Work out the finished part from the listing and answer in its coordinate system (mm). A direction names the side the tool comes from. Give positions to 0.01 mm unless a question says otherwise; leave off trailing zeros. Write each loop counter-clockwise with the first axis right and the second up, starting at its lowest first coordinate (ties: lowest second). Pieces come first, ordered by that corner, then holes.
1) A tool of negligible diameter and unlimited length cuts with its end or side. For faces 5 (the face through (49, 166, 5.5)), 6 (the face through (110, 170, 3)), 7 (the face through (-10, 170, 3)), from which of +Z, -Z, +X, -X, +Y, -Y can it reach the whole face along a straight path? Write none if from no direction.
2) Find section D-D (x = 18). Determine the outline of the cut face in (y, z), plus the area to 3 significant figures.
3) Find section B-B (y = 176.5). Determine the outline of the cut face in (x, z), plus the area to 3 significant figures.
4) Straight lines are drawn through the part: probe 1 along Y at (x, z) = (105, 2.95); probe 2 along X at (y, z) = (186, 1.65); probe 3 along X at (y, z) = (183, 3.4). For each, find the intervals that lie inside material, in ascending order.
5) Find section C-C (x = 50). Determine the outline of the cut face in (y, z).
6) Find section A-A (z = 3.95). Determine the outline of the cut face in (x, y), plus the area to 3 significant figures.
7) Determine the mould class of faces 1 (the face through (49, 166, 0)), 2 (the face through (100, 188, 3)), 3 (the face through (50.82, 170.01, 2.71)), 4 (the face through (-20, 160, 3)) for opening direction X: pulls with the +X half, pulls with the -X half, needs draft (parallel to the pull), parting line crosses it, or undercut.
8) Given pin 1 Ø1.5 at (x, y) = (83.5, 162.5) entering from -Z; pin 2 Ø1.5 at (y, z) = (177, 1) entering from -X, each flat-ended and moving along its own axis, determine where each tip first touches the part or whether it passes through.
Autodesk Inventor part; units mm, degrees
ref_plane "YZ Plane" through (0, 0, 0) normal (1, 0, 0) x (0, 1, 0)
ref_plane "XZ Plane" through (0, 0, 0) normal (0, 1, 0) x (-1, 0, 0)
ref_plane "XY Plane" through (0, 0, 0) normal (0, 0, 1) x (1, 0, 0)
sketch "Sketch1" plane through (0, 0, 0) normal (0, 0, 1) x (1, 0, 0)
  line L0 (0, 170) -> (100, 170)
  circle A0 centre (50, 207.5) radius 37.5
  line L1 (100, 150) -> (0, 150)
  line L2 (120, 170) -> (-20, 170)
  line L3 (100, 170) -> (100, 207.5)
  line L4 (100, 207.5) -> (87.5, 207.5)
  line L5 (0, 170) -> (0, 207.5)
  line L6 (0, 207.5) -> (12.5, 207.5)
  line L7 (-20, 170) -> (-20, 150)
  line L8 (-20, 150) -> (0, 150)
  line L9 (100, 150) -> (120, 150)
  line L10 (120, 150) -> (120, 170)
  point P0 (0, 0)
  dimension "d0" = 75
  dimension "d1" = 140
extrude "Extrusion1" add sketch "Sketch1" along normal blind 5.5 contours L5 L6 A0 L0 | L0 L2 L10 L9 L1 L8 L7 | A0 L4 L3 L0
properties part number "anillo5"
Results:
1. face 5: +Z, +X, -X, +Y, -Y
1. face 6: +Z, -Z, +X, +Y
1. face 7: +Z, -Z, -X, +Y
2. outline: (150, 0) - (187.95, 0) - (187.95, 5.5) - (150, 5.5) - close
2. area: 209 mm2
3. outline: (0, 0) - (28.9, 0) - (28.9, 5.5) - (0, 5.5) - close; (71.1, 0) - (100, 0) - (100, 5.5) - (71.1, 5.5) - close
3. area: 318 mm2
4. probe 1: y = 150 to 170
4. probe 2: x = 0 to 19.28, 80.72 to 100
4. probe 3: x = 0 to 21.61, 78.39 to 100
5. outline: (150, 0) - (170, 0) - (170, 5.5) - (150, 5.5) - close
6. outline: (-20, 150) - (120, 150) - (120, 170) - (100, 170) - (100, 207.5) - (87.5, 207.5) arc R37.5 cw to (12.5, 207.5) - (0, 207.5) - (0, 170) - (-20, 170) - close
6. area: 4,340 mm2
7. face 1: needs draft
7. face 2: pulls with the +X half
7. face 3: undercut
7. face 4: pulls with the -X half
8. pin 1: stops at z = 0
8. pin 2: stops at x = 0
